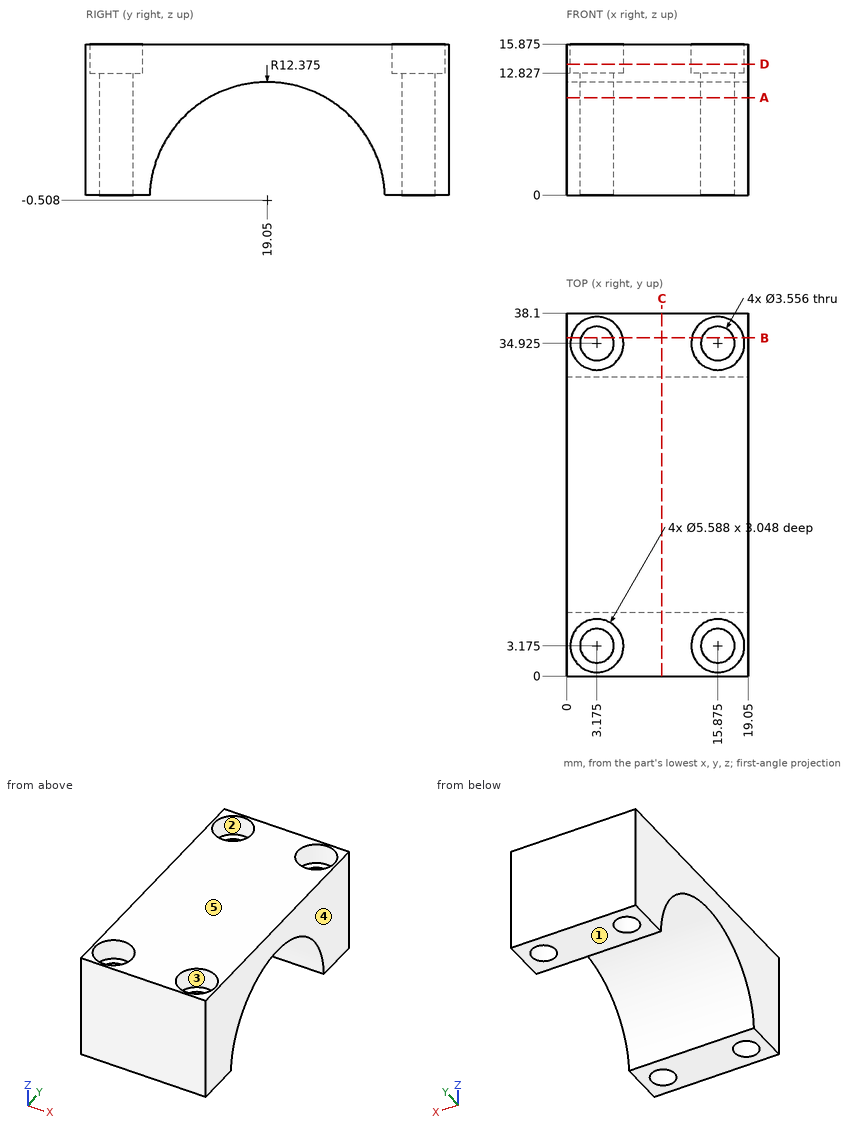
Drawing for the job (mm, zero at the part's lowest x, y, z). A direction names the side the tool comes from. Give positions to 0.01 mm unless a question says otherwise; leave off trailing zeros. Order: outer loops, then holes, each group sorted by start corner. A loop starts at its lowest first (then second) coordinate and runs counter-clockwise, first axis right, second up. Notation, with made-up numbers: M -20.5,-23 L -5.5,-23 A8 cw -5.5,-15 Z; hole C -34,-28 d11. An arc over 180 degrees is marked long. Write item = value, one per line. Start each with the question number.
(1) Slice it at D-D on z = 13.75. Write the cut outline in (x, y) (3 decimals), plus the area to 3 significant figures.
(2) Slice it at C-C on x = 10. Write the cut outline in (y, z) (3 decimals), plus the area to 3 significant figures.
(3) Slice it at B-B on y = 35.5. Write the cut outline in (x, z) (3 decimals).
(4) Two-plate mould, pull along X, no slides. Class the marked faces 3, 4 and 5: released by +X, released by -X, zero draft, split by the parting line, or undercut.
(5) Pin check, flat tips, straight feed: pin 1 Ø4 at (x, y) = (8, 22.5) entering from -Z; pin 2 Ø1.5 at (x, y) = (6, 8.5) entering from -Z; pin 3 Ø4.5 at (x, y) = (3.5, 35) entering from +Z. Stop position of each tip, or through.
(6) Which spindle directions (+Z, -Z, +X, -X, +Y, -Y) get a long thin tool onto all of the face, cutting with end or side? Do the marked faces 1 and 2. Say none if no direction does.
(7) Slice it at A-A on z = 10.25. Write the cut outline in (x, y) (3 decimals), plus the area to 3 significant figures.
(8) Probe L1, parallel to X at y = 2, z = 3.75; L2, parallel to Z at x = 5.5, y = 33.5; L3, parallel to Y at x = 5.5, z = 1. List the from-to ranges inside material, lowest first. Write a range as [from, to].
Responses:
q1.outline = M 0,0 L 19.05,0 L 19.05,38.1 L 0,38.1 Z; hole C 3.175,3.175 d5.588; hole C 3.175,34.925 d5.588; hole C 15.875,3.175 d5.588; hole C 15.875,34.925 d5.588
q1.area = 628 mm2
q2.outline = M 0,0 L 6.685,0 A12.375 cw 31.415,0 L 38.1,0 L 38.1,15.875 L 0,15.875 Z
q2.area = 377 mm2
q3.outline = M 0,0 L 1.493,0 L 1.493,12.827 L 0.441,12.827 L 0.441,15.875 L 0,15.875 Z; M 4.857,0 L 14.193,0 L 14.193,12.827 L 13.141,12.827 L 13.141,15.875 L 5.909,15.875 L 5.909,12.827 L 4.857,12.827 Z; M 17.557,0 L 19.05,0 L 19.05,15.875 L 18.609,15.875 L 18.609,12.827 L 17.557,12.827 Z
q4.face_3 = undercut
q4.face_4 = released by +X
q4.face_5 = zero draft
q5.pin_1 = 10.6
q5.pin_2 = 4.54
q5.pin_3 = 12.83
q6.face_1 = -Z, +X, -X, +Y, -Y
q6.face_2 = +Z
q7.outline = M 0,0 L 19.05,0 L 19.05,12.934 L 0,12.934 Z; M 0,25.166 L 19.05,25.166 L 19.05,38.1 L 0,38.1 Z; hole C 3.175,3.175 d3.556; hole C 3.175,34.925 d3.556; hole C 15.875,3.175 d3.556; hole C 15.875,34.925 d3.556
q7.area = 453 mm2
q8.L1 = [0, 1.84], [4.51, 14.54], [17.21, 19.05]
q8.L2 = [0, 12.83]
q8.L3 = [0, 6.77], [31.33, 38.1]
